The model under review builds one solid part; all positions refer to its coordinate system, in mm. Face numbers are marked on the shaded views. A direction names the side the tool comes from. Round coordinates to 2 decimals unless told otherwise and drop trailing zeros. Order: outer loops, then holes, each group sorted by start corner. A loop starts at its lowest first (then second) coordinate and runs counter-clockwise, first axis right, second up.
1) Machinability: for the marked faces 1 and 2, which of the approach directions +Z, -Z, +X, -X, +Y, -Y give a long, thin tool a straight path to every point of the face, cutting with its end or side? Answer none if there is none.
2) Clearance check with flat-ended pins moving along their axes: P1, Ø1.1, axis at y = 2, z = 2, coming from the -X side; P2, Ø1, axis at y = -11.5, z = 2, coming from the -X side; P3, Ø3, axis at x = -0.5, y = -4, coming from the +Z side; P4, Ø2, axis at x = -4.5, z = 1, coming from the -Y side. State where each tip first meets the part, or that it passes through.
3) Consider section C-C (x = 2.75). Give the boundary of the cut face in (y, z).
4) Consider section D-D (z = 4.6). Give the boundary of the cut face in (x, y), then the cut area to 3 significant figures.
5) Consider section A-A (z = 1.75). Give the boundary of the cut face in (x, y).
6) Consider section B-B (y = -7.5). Give the boundary of the cut face in (x, z), then the cut area to 3 significant figures.
7) To check wall thickness, follow L1, parallel to X at y = -9.25, z = 1.75; L2, parallel to Z at x = -2.75, y = -12.25; L3, parallel to X at y = -15, z = 2.5. State the ranges of each line that lie inside material, in increasing order.
8) Mouldability with a two-part tool opening along Z and no side actions: class the marked faces 3, 4 and 5 as pulls with the +Z half, pulls with the -Z half, needs draft (parallel to the pull), parting line crosses it, or undercut.
from build123d import *

# Parameters (mm, degrees)
F1_DEPTH      = 3.5
F2_R          = 1.75
F2_R_2        = 1.25
F3_DEPTH      = 9.6
F5_DEPTH      = 3.501
F6_W          = 1.2
F6_H          = 4
F7_DEPTH      = 2.2
F7_DEPTH_BACK = 0.5


with BuildPart() as f1:
    # F0 (on Top) → F1 (new body)
    with BuildSketch(Plane.XY):
        Polygon((0, 2.7), (-5.5, 2.7), (-8.75, 0), (-8.75, -4.2), (-5.5, -6.9), (0, -6.9), (3.25, -4.2), (3.25, 0), align=None)
    extrude(amount=F1_DEPTH)

    # F2 (on face) → F3 (join)
    with BuildSketch(Plane.XZ.offset(6.9)):
        with Locations((-2.75, 1.75)):
            Circle(F2_R)
        with Locations((-2.75, 1.75)):
            Circle(F2_R_2, mode=Mode.SUBTRACT)
    extrude(amount=F3_DEPTH)

    # F4 (on face) → F5 (cut, through all)
    with BuildSketch(Plane.XY.offset(3.5)):
        Polygon((-1.45, 2.7), (-4.05, 2.7), (-4.05, 1.7), (-4.7, 1.7), (-4.7, 0.3), (-0.8, 0.3), (-0.8, 1.7), (-1.45, 1.7), align=None)
    extrude(amount=-F5_DEPTH, mode=Mode.SUBTRACT)

    # F6 (on face) → F7 (join, two sides)
    with BuildSketch(Plane.XY.offset(3.5)) as f7_sk:
        with Locations((-2.75, -14.5)):
            Rectangle(F6_W, F6_H)
    extrude(amount=F7_DEPTH)
    extrude(f7_sk.sketch, amount=-F7_DEPTH_BACK)


solid = f1.part
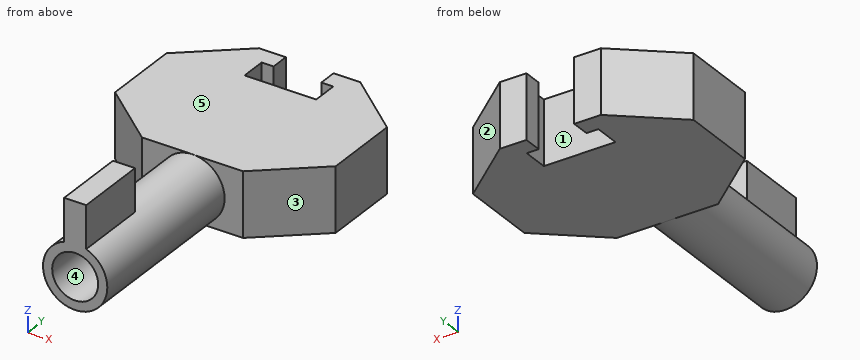
Answer below:
1. face 1: +Z, -Z
1. face 2: +Z, -Z, +X, +Y
2. P1: stops at x = -7
2. P2: stops at x = -4.5
2. P3: stops at z = 3.5
2. P4: stops at y = -16.5
3. outline: (-4.62, 0) - (0.42, 0) - (0.42, 3.5) - (-4.62, 3.5) - close
4. outline: (-3.35, -16.5) - (-2.15, -16.5) - (-2.15, -12.5) - (-3.35, -12.5) - close
4. area: 4.80 mm2
5. outline: (-8.75, -4.2) - (-5.5, -6.9) - (-4.5, -6.9) - (-4.5, -16.5) - (-4, -16.5) - (-4, -6.9) - (-1.5, -6.9) - (-1.5, -16.5) - (-1, -16.5) - (-1, -6.9) - (0, -6.9) - (3.25, -4.2) - (3.25, 0) - (0, 2.7) - (-1.45, 2.7) - (-1.45, 1.7) - (-0.8, 1.7) - (-0.8, 0.3) - (-4.7, 0.3) - (-4.7, 1.7) - (-4.05, 1.7) - (-4.05, 2.7) - (-5.5, 2.7) - (-8.75, 0) - close
6. outline: circle Ø3.5 at (-2.75, 1.75); hole circle Ø2.5 at (-2.75, 1.75)
6. area: 4.71 mm2
7. L1: x = -4.5 to -4, -1.5 to -1
7. L2: z = 0 to 0.5, 3 to 3.5
7. L3: x = -4.33 to -3.75, -1.75 to -1.17
8. face 3: needs draft
8. face 4: undercut
8. face 5: pulls with the +Z half
